Could you check a few things on this drawing? It's one solid part, dimensions in mm from its lowest x, y, z. A direction names the side the tool comes from. Give positions to 0.01 mm unless a question says otherwise; leave off trailing zeros. Order: outer loops, then holes, each group sorted by start corner. A loop starts at its lowest first (then second) coordinate and runs counter-clockwise, first axis right, second up. Notation, with made-up numbers: (40.5, 82.5) - (83.5, 82.5) arc R11 cw to (83.5, 92.5) - close; hole circle Ø11 at (74, 86.5). An arc over 180 degrees is marked (long way). One line per question, with ' | ' between items. Start each with the question number.
1. I need wall thicknesses on probe 1 along X at (y, z) = (3.75, 14); probe 2 along Z at (x, y) = (14, 4); probe 3 along Z at (x, y) = (3, 6). Which ranges of each line are inside material? Lowest first, please. Write a range as from..to.
2. For P1, Ø5, axis at y = 4.5, z = 25, coming from the -X side; P2, Ø4, axis at x = 14, z = 25, coming from the +Y side (1 decimal); P3, Ø3.5, axis at x = 3, z = 14, coming from the +Y side (1 decimal); P4, Ø2.5, axis at x = 14, z = 3, coming from the +Y side, each with a flat end and sliding along its axis, tell me the tip position at first contact or that it passes through.
3. Which directions (+Z, -Z, +X, -X, +Y, -Y) give clear straight access to the entire face, cutting with the end or side of a thin tool? Please do the marked faces 4 and 5.
4. Imagine slicing it at D-D (z = 14). Give the number of separate pieces and of enclosed holes in the cut face.
5. If we mould it in two halves opening along Z, with no side actions, what happens to the marked faces 1, 2 and 3? For each: released by +Z, released by -Z, zero draft, split by the parting line, or undercut.
6. Imagine slicing it at C-C (y = 3.5). Please give me the cut outline in (x, z).
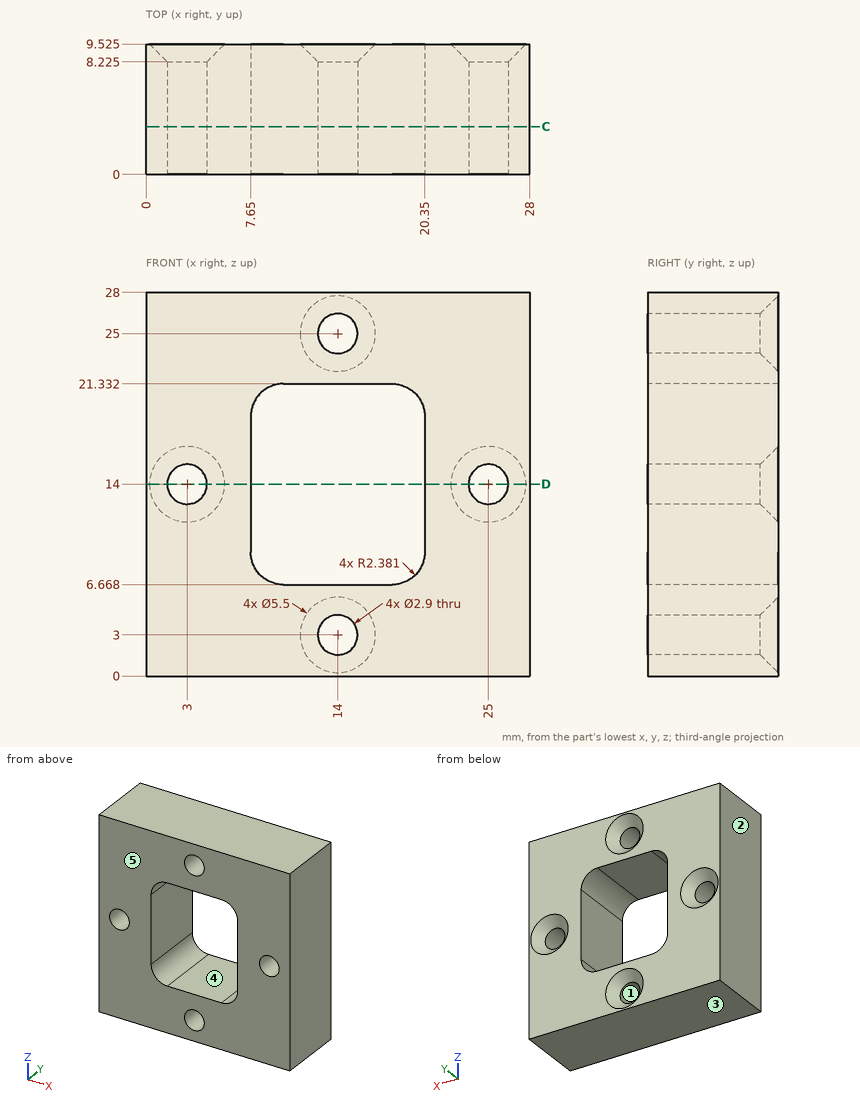
Results found:
1) probe 1: x = 0..1.55, 4.45..7.65, 20.35..23.55, 26.45..28 | probe 2: z = 0..1.55, 4.45..6.67, 21.33..23.55, 26.45..28 | probe 3: z = 0..12.55, 15.45..28
2) P1: stops at x = 0 | P2: stops at y = 8.8 | P3: stops at y = 8.5 | P4: passes through
3) face 4: +Y, -Y | face 5: +Z, -Z, +X, -X, -Y
4) separate pieces: 4 | enclosed holes: 0
5) face 1: undercut | face 2: zero draft | face 3: released by -Z
6) outline: (0, 0) - (28, 0) - (28, 28) - (0, 28) - close; hole circle Ø2.9 at (3, 14); hole (7.65, 9.05) arc R2.38 ccw to (10.03, 6.67) - (17.97, 6.67) arc R2.38 ccw to (20.35, 9.05) - (20.35, 18.95) arc R2.38 ccw to (17.97, 21.33) - (10.03, 21.33) arc R2.38 ccw to (7.65, 18.95) - close; hole circle Ø2.9 at (14, 3); hole circle Ø2.9 at (14, 25); hole circle Ø2.9 at (25, 14)
